Part model, mm, in its own coordinate system. Face numbers are marked on the shaded views. Coordinates: 2 decimals unless noted, no trailing zeros. Loops run counter-clockwise (first coordinate to the right, second up) from the corner with the lowest first, then second, coordinate; pieces in that order, holes last. Notation, with made-up numbers: (10.25, 52.25) - (64.25, 52.25) arc R6 ccw to (64.25, 61.25) - close; hole circle Ø2 at (79.25, 42.25). An arc over 180 degrees is marked (long way). Use a Markdown table: item, result. Add a question column.
1. Band-saw the part on B-B, the plane x = 14. Give the cut face in (y, z), plus the area to 3 significant figures.
2. Band-saw the part on A-A, the plane y = 24.5. Give the cut face in (x, z).
3. Wall check: probe 1 along Y at (x, z) = (19, 21.1); probe 2 along X at (y, z) = (32, 21.65); probe 3 along X at (y, z) = (37, 19.9). Give the ranges that are in metal, low to high. Write a range as [from, to].
4. Drop flat-ended pins along their axis: pin 1 (0.8 mm diameter, centred on y = -2.5, z = 21, fed in from +X); pin 2 (2 mm diameter, centred on y = 41.5, z = 21, fed in from -X); pin 3 (0.5 mm diameter, centred on y = -2, z = 21, fed in from -X); pin 4 (1.3 mm diameter, centred on x = -7.5, y = 40, fed in from +Z). Give the stop position or say it passes through.
5. Pull direction X, two halves, no side cores. Call the marked faces 1, 2 and 3: pulls with the +X half, pulls with the -X half, needs draft (parallel to the pull), parting line crosses it, or undercut.
from build123d import *

# Parameters (mm, degrees)
SKETCH033_R     = 1.1
PAD017_DEPTH    = 4.8
POCKET009_DEPTH = 2.5
POCKET010_DEPTH = 3
CHAMFER011_SIZE = 1.5
SKETCH040_R     = 6.75
POCKET014_DEPTH = 2


with BuildPart() as part:
    # Sketch033 → Pad017 (new body)
    with BuildSketch(Plane.XY):
        with BuildLine():
            Line((0, 10), (0, 42))
            ThreePointArc((5.5, 50.930286), (1.485307, 47.244044), (0, 42))
            Line((5.5, 50.930286), (5.5, 52))
            Line((5.5, 52), (77.5, 52))
            Line((77.5, 52), (77.5, 50.930286))
            ThreePointArc((83, 42), (81.514693, 47.244044), (77.5, 50.930286))
            Line((83, 42), (83, 10))
            ThreePointArc((77.5, 1.069714), (81.514693, 4.755956), (83, 10))
            Line((77.5, 1.069714), (77.5, 0))
            Line((5.5, 0), (77.5, 0))
            Line((5.5, 1.069714), (5.5, 0))
            ThreePointArc((0, 10), (1.485307, 4.755956), (5.5, 1.069714))
        make_face()
        with Locations((5.5, 46.5)):
            Circle(SKETCH033_R, mode=Mode.SUBTRACT)
        with Locations((77.5, 46.5)):
            Circle(SKETCH033_R, mode=Mode.SUBTRACT)
        with Locations((5.5, 5.5)):
            Circle(SKETCH033_R, mode=Mode.SUBTRACT)
        with Locations((77.5, 5.5)):
            Circle(SKETCH033_R, mode=Mode.SUBTRACT)
    extrude(amount=PAD017_DEPTH)

    # Sketch034 → Pocket009 (cut)
    with BuildSketch(Plane.XY):
        with BuildLine():
            Line((9.5, 50.3), (73.5, 50.3))
            ThreePointArc((74.8, 49), (74.419239, 49.919239), (73.5, 50.3))
            Line((74.8, 46.5), (74.8, 49))
            ThreePointArc((74.8, 46.5), (75.590812, 44.590812), (77.5, 43.8))
            Line((80, 43.8), (77.5, 43.8))
            ThreePointArc((81.3, 42.5), (80.919239, 43.419239), (80, 43.8))
            Line((81.3, 42.5), (81.3, 9.5))
            ThreePointArc((80, 8.2), (80.919239, 8.580761), (81.3, 9.5))
            Line((77.5, 8.2), (80, 8.2))
            ThreePointArc((77.5, 8.2), (75.590812, 7.409188), (74.8, 5.5))
            Line((74.8, 3), (74.8, 5.5))
            ThreePointArc((73.5, 1.7), (74.419239, 2.080761), (74.8, 3))
            Line((73.5, 1.7), (9.5, 1.7))
            ThreePointArc((8.2, 3), (8.580761, 2.080761), (9.5, 1.7))
            Line((8.2, 5.5), (8.2, 3))
            ThreePointArc((8.2, 5.5), (7.409188, 7.409188), (5.5, 8.2))
            Line((3, 8.2), (5.5, 8.2))
            ThreePointArc((1.7, 9.5), (2.080761, 8.580761), (3, 8.2))
            Line((1.7, 9.5), (1.7, 42.5))
            ThreePointArc((3, 43.8), (2.080761, 43.419239), (1.7, 42.5))
            Line((5.5, 43.8), (3, 43.8))
            ThreePointArc((5.5, 43.8), (7.409188, 44.590812), (8.2, 46.5))
            Line((8.2, 49), (8.2, 46.5))
            ThreePointArc((9.5, 50.3), (8.580761, 49.919239), (8.2, 49))
        make_face()
        with BuildLine():
            Line((10.3, 48.7), (72.7, 48.7))
            ThreePointArc((73.2, 48.2), (73.053553, 48.553553), (72.7, 48.7))
            Line((73.2, 46.5), (73.2, 48.2))
            ThreePointArc((73.2, 46.5), (74.459441, 43.459441), (77.5, 42.2))
            Line((79.2, 42.2), (77.5, 42.2))
            ThreePointArc((79.7, 41.7), (79.553553, 42.053553), (79.2, 42.2))
            Line((79.7, 41.7), (79.7, 10.3))
            ThreePointArc((79.2, 9.8), (79.553553, 9.946447), (79.7, 10.3))
            Line((77.5, 9.8), (79.2, 9.8))
            ThreePointArc((77.5, 9.8), (74.459441, 8.540559), (73.2, 5.5))
            Line((73.2, 3.8), (73.2, 5.5))
            ThreePointArc((72.7, 3.3), (73.053553, 3.446447), (73.2, 3.8))
            Line((72.7, 3.3), (10.3, 3.3))
            ThreePointArc((9.8, 3.8), (9.946447, 3.446447), (10.3, 3.3))
            Line((9.8, 3.8), (9.8, 5.5))
            ThreePointArc((9.8, 5.5), (8.540559, 8.540559), (5.5, 9.8))
            Line((5.5, 9.8), (3.8, 9.8))
            ThreePointArc((3.3, 10.3), (3.446447, 9.946447), (3.8, 9.8))
            Line((3.3, 10.3), (3.3, 41.7))
            ThreePointArc((3.8, 42.2), (3.446447, 42.053553), (3.3, 41.7))
            Line((5.5, 42.2), (3.8, 42.2))
            ThreePointArc((5.5, 42.2), (8.540559, 43.459441), (9.8, 46.5))
            Line((9.8, 48.2), (9.8, 46.5))
            ThreePointArc((10.3, 48.7), (9.946447, 48.553553), (9.8, 48.2))
        make_face(mode=Mode.SUBTRACT)
    extrude(amount=POCKET009_DEPTH, mode=Mode.SUBTRACT)

    # Sketch035 → Pocket010 (cut)
    with BuildSketch(Plane.XY):
        with BuildLine():
            Line((11.3, 47.7), (71.7, 47.7))
            ThreePointArc((72.2, 47.2), (72.053553, 47.553553), (71.7, 47.7))
            Line((72.2, 46.5), (72.2, 47.2))
            ThreePointArc((72.2, 46.5), (73.752334, 42.752334), (77.5, 41.2))
            Line((78.2, 41.2), (77.5, 41.2))
            ThreePointArc((78.7, 40.7), (78.553553, 41.053553), (78.2, 41.2))
            Line((78.7, 40.7), (78.7, 11.3))
            ThreePointArc((78.2, 10.8), (78.553553, 10.946447), (78.7, 11.3))
            Line((77.5, 10.8), (78.2, 10.8))
            ThreePointArc((77.5, 10.8), (73.752334, 9.247666), (72.2, 5.5))
            Line((72.2, 4.8), (72.2, 5.5))
            ThreePointArc((71.7, 4.3), (72.053553, 4.446447), (72.2, 4.8))
            Line((71.7, 4.3), (11.3, 4.3))
            ThreePointArc((10.8, 4.8), (10.946447, 4.446447), (11.3, 4.3))
            Line((10.8, 5.5), (10.8, 4.8))
            ThreePointArc((10.8, 5.5), (9.247666, 9.247666), (5.5, 10.8))
            Line((4.8, 10.8), (5.5, 10.8))
            ThreePointArc((4.3, 11.3), (4.446447, 10.946447), (4.8, 10.8))
            Line((4.3, 11.3), (4.3, 40.7))
            ThreePointArc((4.8, 41.2), (4.446447, 41.053553), (4.3, 40.7))
            Line((5.5, 41.2), (4.8, 41.2))
            ThreePointArc((5.5, 41.2), (9.247666, 42.752334), (10.8, 46.5))
            Line((10.8, 47.2), (10.8, 46.5))
            ThreePointArc((11.3, 47.7), (10.946447, 47.553553), (10.8, 47.2))
        make_face()
    extrude(amount=POCKET010_DEPTH, mode=Mode.SUBTRACT)

    # Chamfer011
    chamfer011_edges = [part.edges().sort_by_distance(p)[0] for p in [
        (76.4, 46.5, 4.8),
        (76.4, 5.5, 4.8),
        (4.4, 5.5, 4.8),
        (4.4, 46.5, 4.8),
    ]]
    chamfer(chamfer011_edges, length=CHAMFER011_SIZE)

    # Sketch040 (on Face79 of Chamfer011) → Pocket014 (cut)
    with BuildSketch(Plane(origin=(78.7, 0, 0), x_dir=(0, -1, 0), z_dir=(-1, 0, 0))):
        with Locations((-25.5, -6)):
            Circle(SKETCH040_R)
    extrude(amount=-POCKET014_DEPTH, mode=Mode.SUBTRACT)


with BuildPart() as part_1:
    # Body009 placement: moved
    add(part.part.moved(Location((-13, -6.5, 19.5))))


solid = part_1.part
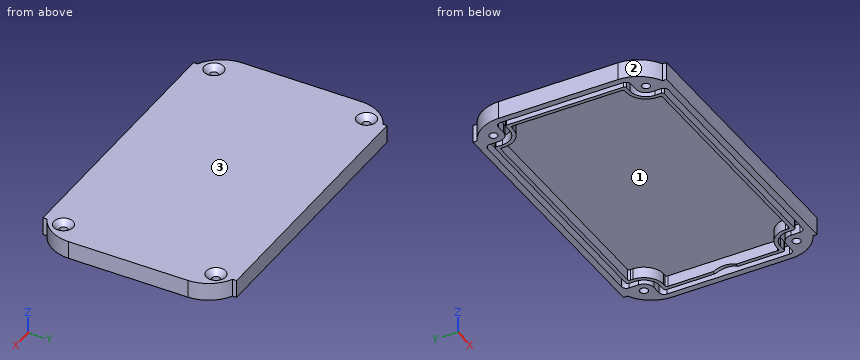
Geometry check:
| question | item | result |
|---|---|---|
| 1 | outline | (-6.5, 19.5) - (-4.8, 19.5) - (-4.8, 22) - (-3.2, 22) - (-3.2, 19.5) - (-2.2, 19.5) - (-2.2, 22.5) - (41.2, 22.5) - (41.2, 19.5) - (42.2, 19.5) - (42.2, 22) - (43.8, 22) - (43.8, 19.5) - (45.5, 19.5) - (45.5, 24.3) - (-6.5, 24.3) - close |
| 1 | area | 111 mm^2 |
| 2 | outline | (-13, 19.5) - (-11.3, 19.5) - (-11.3, 22) - (-9.7, 22) - (-9.7, 19.5) - (-8.7, 19.5) - (-8.7, 22.5) - (65.7, 22.5) - (65.7, 19.5) - (66.7, 19.5) - (66.7, 22) - (68.3, 22) - (68.3, 19.5) - (70, 19.5) - (70, 24.3) - (-13, 24.3) - close |
| 3 | probe 1 | y = [-6.5, -4.8], [-3.2, -2.2], [41.2, 42.2], [43.8, 45.5] |
| 3 | probe 2 | x = [-13, -11.3], [-9.7, -8.7], [65.7, 66.7], [68.3, 70] |
| 3 | probe 3 | x = [-12.89, -10.83], [-4.42, -3.13], [60.13, 61.42], [67.83, 69.89] |
| 4 | pin 1 | stops at x = 68.28 |
| 4 | pin 2 | stops at x = -11.66 |
| 4 | pin 3 | stops at x = -11.51 |
| 4 | pin 4 | passes through |
| 5 | face 1 | undercut |
| 5 | face 2 | pulls with the -X half |
| 5 | face 3 | needs draft |
